Autodesk Inventor part; units mm, degrees
ref_plane "Work Plane1" through (-2.0787, -11.43, 0) normal (0, 1, 0) x (1, 0, 0)
ref_plane "Work Plane2" through (-2.0787, 11.43, 0) normal (0, -1, 0) x (1, 0, 0)
ref_plane "YZ Plane" through (0, 0, 0) normal (1, 0, 0) x (0, 1, 0)
sketch "Sketch1" plane through (0, 0, 0) normal (0, 0, 1) x (1, 0, 0)
  line L0 (7.3323, 0) -> (3.6662, -6.35)
  line L1 (3.6662, -6.35) -> (-3.6662, -6.35)
  line L2 (-3.6662, -6.35) -> (-7.3323, 0)
  line L3 (-7.3323, 0) -> (-3.6662, 6.35)
  line L4 (-3.6662, 6.35) -> (3.6662, 6.35)
  line L5 (3.6662, 6.35) -> (7.3323, 0)
  circle A0 centre (0, 0) radius 12.7
  circle A1 centre (44.45, 0) radius 6.35
  line L6 (45.3571, 6.2849) -> (1.8143, 12.5697)
  line L7 (45.3571, -6.2849) -> (1.8143, -12.5697)
  line L8 (0, 0) -> (64.5311, 0) construction
  dimension "d0" = 12.7
  dimension "d1" = 25.4
  dimension "d2" = 44.45
  dimension "d3" = 12.7
extrude "Extrusion1" add sketch "Sketch1" along normal blind 6.35
hole "Hole1" at (44.45, 0, 0) direction (0, 0, 1) diameter 3.9624 depth 13.6144
hole "Hole2" at (3.6662, -6.35, 0) at (7.3323, 0, 0) at (3.6662, 6.35, 0) at (-3.6662, 6.35, 0) at (-7.3323, 0, 0) at (-3.6662, -6.35, 0) direction (0, 0, 1) diameter 3.175 depth 13.6144
sketch "Sketch2" plane through (0, 0, 6.35) normal (0, 0, 1) x (1, 0, 0)
  arc A0 (1.8143, 12.5697) -> (1.8143, -12.5697) centre (0, 0) ccw
  circle A1 centre (0, 0) radius 12.7
  line L0 (-2.0787, 6.35) -> (2.0787, 6.35)
  arc A2 (4.4599, 4.9752) -> (2.0787, 6.35) centre (3.6662, 6.35) ccw
  arc A3 (-2.0787, 6.35) -> (-4.4599, 4.9752) centre (-3.6662, 6.35) ccw
  line L1 (-6.5386, 1.3748) -> (-4.4599, 4.9752)
  arc A4 (-6.5386, 1.3748) -> (-6.5386, -1.3748) centre (-7.3323, 0) ccw
  line L2 (-4.4599, -4.9752) -> (-6.5386, -1.3748)
  arc A5 (-4.4599, -4.9752) -> (-2.0787, -6.35) centre (-3.6662, -6.35) ccw
  line L3 (2.0787, -6.35) -> (-2.0787, -6.35)
  arc A6 (2.0787, -6.35) -> (4.4599, -4.9752) centre (3.6662, -6.35) ccw
  line L4 (6.5386, -1.3748) -> (4.4599, -4.9752)
  arc A7 (6.5386, -1.3748) -> (6.5386, 1.3748) centre (7.3323, 0) ccw
  line L5 (4.4599, 4.9752) -> (6.5386, 1.3748)
  point P0 (1.8143, -12.5697)
extrude "Extrusion2" add sketch "Sketch2" along normal blind 12.7
chamfer "Chamfer1" [suppressed]
ref_plane "Work Plane1" through (-2.0787, -11.43, 0) normal (0, 1, 0) x (1, 0, 0)
sketch "Sketch3" plane through (-2.0787, -11.43, 0) normal (0, 1, 0) x (1, 0, 0)
  line L0 (-10.6213, 0) -> (3.893, 0)
  line L1 (-10.6213, -19.05) -> (14.7787, -19.05)
  line L2 (-10.6213, 0) -> (14.7787, 0)
  line L3 (14.7787, 0) -> (14.7787, -19.05)
  line L4 (14.7787, -19.05) -> (-10.6213, -19.05)
  line L5 (-10.6213, -19.05) -> (-10.6213, 0)
  point P0 (2.0787, 0)
  point P1 (-10.6213, -19.05)
extrude "Extrusion3" cut sketch "Sketch3" against normal through all
ref_plane "Work Plane2" through (-2.0787, 11.43, 0) normal (0, -1, 0) x (1, 0, 0)
sketch "Sketch4" plane through (-2.0787, 11.43, 0) normal (0, -1, 0) x (1, 0, 0)
  line L0 (3.893, 0) -> (-10.6213, 0)
  line L1 (14.7787, 19.05) -> (-10.6213, 19.05)
  line L2 (-10.6213, 0) -> (14.7787, 0)
  line L3 (14.7787, 0) -> (14.7787, 19.05)
  line L4 (14.7787, 19.05) -> (-10.6213, 19.05)
  line L5 (-10.6213, 19.05) -> (-10.6213, 0)
  point P0 (2.0787, 0)
  point P1 (-3.4571, 0)
  point P2 (7.6145, 19.05)
  point P3 (-3.4571, 19.05)
  point P4 (-10.6213, 19.05)
extrude "Extrusion4" cut sketch "Sketch4" against normal through all
properties part number "Lower Linkage"
Design review of the part built by this model. Coordinates are the model's own, in mm. A direction names the side the tool comes from. Coordinates: 2 decimals unless noted, no trailing zeros. Order: outer loops, then holes, each group sorted by start corner. A loop starts at its lowest first (then second) coordinate and runs counter-clockwise, first axis right, second up.
Item 1: Take a section at B-B, the plane y = 0.25. Count the separate pieces of the cut face and the enclosed holes in it, then the cut area to 3 significant figures.
Item 2: For pin 1 Ø2.5 at (x, y) = (3.67, -6.35) entering from +Z; pin 2 Ø1.5 at (y, z) = (-8.5, 14) entering from +X; pin 3 Ø3 at (x, z) = (10, 9) entering from -Y; pin 4 Ø5 at (y, z) = (-4.5, 6) entering from +X, all flat-tipped, find the tip position at first contact; note any pin that passes through.
Item 3: For line 1 (Y direction, x = 5.5, z = 4.5); line 2 (Y direction, x = -1.5, z = 12.5); line 3 (X direction, y = -7, z = 15), list the stretches that pass through material, from the lowest coordinate up.
Item 4: For faces 1 (the flat face through (0, 11.43, 10)), 2 (the flat face through (5.485, 3.2, 12.611)), list the 3-axis set-ups (+Z, -Z, +X, -X, +Y, -Y) from which the entire face can be reached by the end or side of a thin tool; tool diameter is ignored.
Item 5: Take a section at C-C, the plane x = 44.45. Write out the cut boundary in (y, z).
Item 6: Take a section at A-A, the plane z = 10.5. Write out the cut boundary in (x, y), then the cut area to 3 significant figures.
Item 7: The part is to be moulded in two halves that separate along Y. For faces 3 (the cylindrical face through (50.8, 0.1, 3.1)), 4 (the flat face through (27.78, 8.82, 3.13)), 5 (the cylindrical face through (-4.419, -7.747, 12.611)), say which applies: pulls with the +Y half, pulls with the -Y half, needs draft (parallel to the pull), parting line crosses it, or undercut.
The answers:
1. separate pieces: 3
1. enclosed holes: 0
1. area: 362 mm2
2. pin 1: passes through
2. pin 2: stops at x = 10.06
2. pin 3: stops at y = -9.44
2. pin 4: stops at x = 50.48
3. line 1: y = -11.43 to -3.17, 3.17 to 11.43
3. line 2: y = -11.43 to -6.35, 6.35 to 11.43
3. line 3: x = -10.6 to -5.11, -2.22 to 2.22, 5.11 to 10.6
4. face 1: +Z, -Z, +X, -X, +Y
4. face 2: +Z, -Z
5. outline: (-6.42, 0) - (-1.98, 0) - (-1.98, 6.35) - (-6.42, 6.35) - close; (1.98, 0) - (6.42, 0) - (6.42, 6.35) - (1.98, 6.35) - close
6. outline: (-5.54, -11.43) - (5.54, -11.43) arc R12.7 ccw to (5.54, 11.43) - (-5.54, 11.43) arc R12.7 ccw to start; hole (-6.54, -1.37) - (-4.46, -4.98) arc R1.59 ccw (long way) to (-2.08, -6.35) - (2.08, -6.35) arc R1.59 ccw (long way) to (4.46, -4.98) - (6.54, -1.37) arc R1.59 ccw (long way) to (6.54, 1.37) - (4.46, 4.98) arc R1.59 ccw (long way) to (2.08, 6.35) - (-2.08, 6.35) arc R1.59 ccw (long way) to (-4.46, 4.98) - (-6.54, 1.37) arc R1.59 ccw (long way) to start
6. area: 316 mm2
7. face 3: parting line crosses it
7. face 4: pulls with the +Y half
7. face 5: undercut
